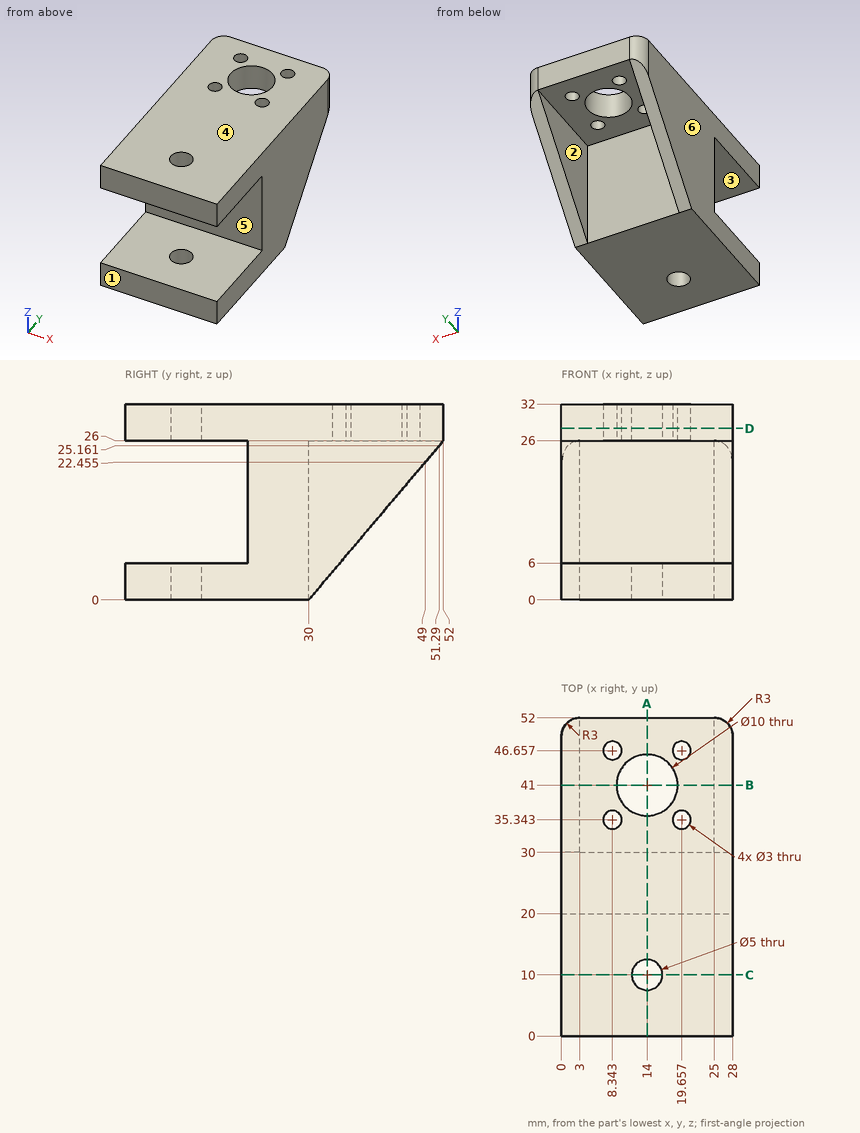
Here's the drawing with two shaded views (mm, measured from the low corner). I have some questions. A direction names the side the tool comes from. Coordinates: 2 decimals unless noted, no trailing zeros. Order: outer loops, then holes, each group sorted by start corner. A loop starts at its lowest first (then second) coordinate and runs counter-clockwise, first axis right, second up.
Q1. Suppose I cut it at D-D on z = 28. Please give me the cut outline in (x, y), and give its area (3 significant figures).
Q2. Which directions (+Z, -Z, +X, -X, +Y, -Y) give clear straight access to the entire face, cutting with the end or side of a thin tool? Please do the marked faces 1, 2 and 3.
Q3. Please list where these lines run through material, in increasing order: L1, parallel to Y at x = 14, z = 27.4; L2, parallel to Z at x = 5, y = 13.5; L3, parallel to Z at x = 15, y = 49.5.
Q4. Suppose I cut it at A-A on x = 14. Please give me the cut outline in (y, z), and give its area (3 significant figures).
Q5. Suppose I cut it at C-C on y = 10. Please give me the cut outline in (x, z), and give its area (3 significant figures).
Q6. Thinking about a two-plate mould opening in Z: for the marked faces 4, 5 and 6, which applies, released by +Z, released by -Z, zero draft, split by the parting line, or undercut?
Q7. Suppose I cut it at B-B on y = 41. Please give me the cut outline in (x, z), and give its area (3 significant figures).
Q8. Will these pins go through, and if not, where does the flat tip stop? pin 1 (3.5 mm diameter, centred on x = 8.34, y = 46.66, fed in from -Z); pin 2 (6 mm diameter, centred on x = 15.5, z = 18.5, fed in from -Y); pin 3 (6 mm diameter, centred on x = 14, y = 41, fed in from -Z); pin 4 (5 mm diameter, centred on x = 3.5, y = 46, fed in from -Z) (1 decimal).
Answer:
1. outline: (0, 0) - (28, 0) - (28, 49) arc R3 ccw to (25, 52) - (3, 52) arc R3 ccw to (0, 49) - close; hole circle Ø3 at (8.34, 35.34); hole circle Ø3 at (8.34, 46.66); hole circle Ø10 at (14, 41); hole circle Ø5 at (14, 10); hole circle Ø3 at (19.66, 35.34); hole circle Ø3 at (19.66, 46.66)
1. area: 1,330 mm2
2. face 1: +Z, -Z, +X, -X, -Y
2. face 2: -Z, +Y
2. face 3: +X, -X, -Y
3. L1: y = 0 to 7.5, 12.5 to 36, 46 to 52
3. L2: z = 0 to 6, 26 to 32
3. L3: z = 26 to 32
4. outline: (0, 0) - (7.5, 0) - (7.5, 6) - (0, 6) - close; (0, 26) - (7.5, 26) - (7.5, 32) - (0, 32) - close; (12.5, 0) - (30, 0) - (30, 26) - (36, 26) - (36, 32) - (12.5, 32) - (12.5, 26) - (20, 26) - (20, 6) - (12.5, 6) - close; (46, 26) - (52, 26) - (52, 32) - (46, 32) - close
4. area: 572 mm2
5. outline: (0, 0) - (11.5, 0) - (11.5, 6) - (0, 6) - close; (0, 26) - (11.5, 26) - (11.5, 32) - (0, 32) - close; (16.5, 0) - (28, 0) - (28, 6) - (16.5, 6) - close; (16.5, 26) - (28, 26) - (28, 32) - (16.5, 32) - close
5. area: 276 mm2
6. face 4: released by +Z
6. face 5: undercut
6. face 6: zero draft
7. outline: (0, 13) - (3, 13) - (3, 26) - (9, 26) - (9, 32) - (0, 32) - close; (19, 26) - (25, 26) - (25, 13) - (28, 13) - (28, 32) - (19, 32) - close
7. area: 186 mm2
8. pin 1: stops at z = 26
8. pin 2: stops at y = 20
8. pin 3: passes through
8. pin 4: stops at z = 16
